Can you work these out from the model? Positions are in its coordinate system, mm. Face numbers are marked on the shaded views. A direction names the side the tool comes from. Coordinates: 2 decimals unless noted, no trailing zeros. Order: outer loops, then holes, each group sorted by start corner. A loop starts at its lowest first (then second) coordinate and runs counter-clockwise, first axis right, second up. Notation, with made-up numbers: M 24.25,58 L 29.25,58 A15 cw 29.25,71 Z; hole C 73,-21 d11. An arc over 180 degrees is marked long. Answer as a JSON object with one key per item and string values.
from build123d import *

# Parameters (mm, degrees)
BASE_FLANGE1_DEPTH = 3.175
EDGE_FLANGE1_DEPTH = 660.4
SKETCH9_R          = 3.175
SKETCH9_R_2        = 14.2875
SKETCH9_R_3        = 4.7625
CUT_EXTRUDE1_DEPTH = 410.020846046
CUT_EXTRUDE2_DEPTH = 410.082455778


# Sheet-metal steps are written as plain solids
with BuildPart() as part:
    # Sketch1 → Base-Flange1 (new body)
    with BuildSketch(Plane(origin=(0, 0, 0), x_dir=(0, 0, -1), z_dir=(1, 0, 0))):
        Polygon((330.2, 0), (-330.2, 0), (-368.3, 38.1), (-368.3, 177.8), (368.3, 177.8), (368.3, 38.1), align=None)
    extrude(amount=-BASE_FLANGE1_DEPTH)

    # Edge-Flange1 section (across the edge) → Edge-Flange1 (add)
    with BuildSketch(Plane(origin=(0, -0.7366, 330.2), x_dir=(0, 1, 0), z_dir=(0, 0, -1))):
        with BuildLine():
            Line((-3.175, 0.7366), (-3.175, 6.35))
            Line((-3.175, 6.35), (0, 6.35))
            Line((0, 6.35), (0, 0.7366))
            ThreePointArc((0, 0.7366), (0.215745145, 0.215745145), (0.7366, 0))
            Line((0.7366, 0), (0.7366, -3.175))
            ThreePointArc((0.7366, -3.175), (-2.029318885, -2.029318885), (-3.175, 0.7366))
        make_face()
    extrude(amount=EDGE_FLANGE1_DEPTH)

    # Sketch9 → Cut-Extrude1 (cut, through all)
    with BuildSketch(Plane(origin=(0, 0, 0), x_dir=(0, 0, -1), z_dir=(1, 0, 0))):
        with Locations((-355.6, 165.1)):
            Circle(SKETCH9_R)
        with Locations((-355.6, 43.360512242)):
            Circle(SKETCH9_R)
        with Locations((-177.8, 165.1)):
            Circle(SKETCH9_R)
        with Locations((0, 165.1)):
            Circle(SKETCH9_R)
        with Locations((-132.489589571, 14.2875)):
            Circle(SKETCH9_R)
        with Locations((132.489589571, 14.2875)):
            Circle(SKETCH9_R)
        with Locations((177.8, 165.1)):
            Circle(SKETCH9_R)
        with Locations((355.6, 165.1)):
            Circle(SKETCH9_R)
        with Locations(Location((355.6, 43.360512242, 0), (0, 0, 180))):
            Circle(SKETCH9_R)
        with Locations((0, 69.85)):
            Circle(SKETCH9_R_2)
        with Locations((-264.979179141, 73.025)):
            Circle(SKETCH9_R_3)
        with Locations((264.979179141, 73.025)):
            Circle(SKETCH9_R_3)
    extrude(amount=-CUT_EXTRUDE1_DEPTH, mode=Mode.SUBTRACT)

    # Sketch10 → Cut-Extrude2 (cut, through all)
    with BuildSketch(Plane.ZY.offset(3.175)):
        with BuildLine():
            Line((-302.426875206, 146.05), (-50.8, 146.05))
            ThreePointArc((-50.8, 146.05), (-41.819743879, 142.330256121), (-38.1, 133.35))
            Line((-38.1, 133.35), (-38.1, 46.0375))
            ThreePointArc((-38.1, 46.0375), (-41.819743879, 37.057243879), (-50.8, 33.3375))
            Line((-50.8, 33.3375), (-143.295855515, 33.3375))
            ThreePointArc((-143.295855515, 33.3375), (-150.12485752, 34.272734895), (-156.450968109, 37.009568376))
            Line((-156.450968109, 37.009568376), (-307.360042429, 128.377025641))
            ThreePointArc((-307.360042429, 128.377025641), (-311.60116212, 139.085875752), (-302.426875206, 146.05))
        make_face()
        with BuildLine():
            Line((38.1, 133.35), (38.1, 46.0375))
            ThreePointArc((38.1, 46.0375), (41.819743879, 37.057243879), (50.8, 33.3375))
            Line((50.8, 33.3375), (143.295855515, 33.3375))
            ThreePointArc((143.295855515, 33.3375), (150.12485752, 34.272734895), (156.450968109, 37.009568376))
            Line((156.450968109, 37.009568376), (307.360042429, 128.377025641))
            ThreePointArc((307.360042429, 128.377025641), (311.60116212, 139.085875752), (302.426875206, 146.05))
            Line((302.426875206, 146.05), (50.8, 146.05))
            ThreePointArc((50.8, 146.05), (41.819743879, 142.330256121), (38.1, 133.35))
        make_face()
    extrude(amount=-CUT_EXTRUDE2_DEPTH, mode=Mode.SUBTRACT)


solid = part.part
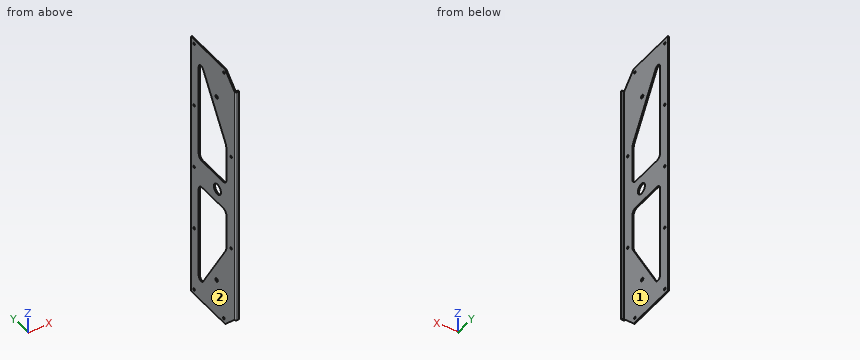
Item 1: I want a section at A-A, the plane z = -210. Write out the boundary of the cut face in (x, y) (3 decimals).
Answers follow:
{"outline": "M -3.175,0 A3.912 ccw 0.737,-3.912 L 6.35,-3.912 L 6.35,-0.737 L 0.737,-0.737 A0.737 cw 0,0 L 0,69.431 L -3.175,69.431 Z; M -3.175,146.05 L 0,146.05 L 0,177.8 L -3.175,177.8 Z"}
Item 2: Which directions (+Z, -Z, +X, -X, +Y, -Y) give clear straight access to the entire face, cutting with the end or side of a thin tool? Please do the marked faces 1 and 2.
Answers follow:
{"face 1": "+Z, -Z, +X, +Y", "face 2": "+Z, -Z, -X, +Y, -Y"}
Item 3: Please list where these lines run through material, in increasing order: line 1 (Y direction, x = -0.9, z = -355.6) (3 decimals); line 2 (Z direction, x = -1.1, y = 165.1) (3 decimals); line 3 (Z direction, x = -2, y = 57).
Answers follow:
{"line 1": "y = 25.4 to 40.186, 46.536 to 161.925, 168.275 to 177.8", "line 2": "z = -368.3 to -358.775, -352.425 to -180.975, -174.625 to -3.175, 3.175 to 174.625, 180.975 to 352.425, 358.775 to 368.3", "line 3": "z = -368.3 to -189.47, -38.1 to -6.25, 6.25 to 38.1, 189.47 to 368.3"}
Item 4: I'm going to push flat-ended pins straight in: pin 1 (2.5 mm diameter, centred on x = -1.5, z = -178.5, fed in from -Y); pin 2 (4 mm diameter, centred on y = 43.36, z = -355.6, fed in from +X); pin 3 (3 mm diameter, centred on x = -1, z = -15, fed in from -Y); pin 4 (2 mm diameter, centred on x = 2.5, y = -3, fed in from +Z). Where does each tip first touch, or does it pass through?
Answers follow:
{"pin 1": "stops at y = -3.79", "pin 2": "passes through", "pin 3": "stops at y = -3.9", "pin 4": "stops at z = 330.2"}
